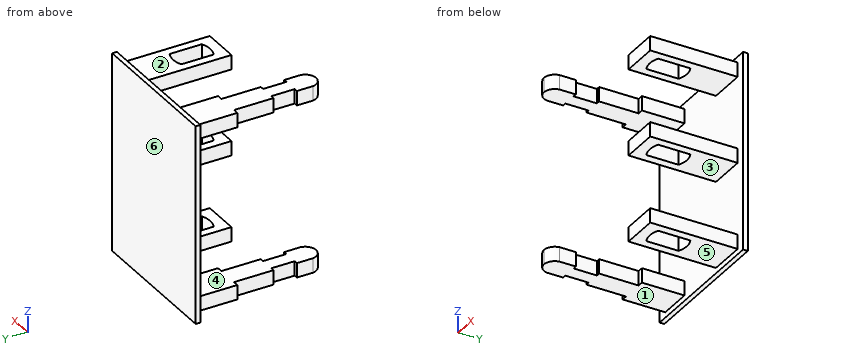
Autodesk Inventor part; units mm, degrees
ref_plane "terminal_to_body_XY" through (0, 0, 0) normal (0, 1, 0) x (1, 0, 0)
ref_plane "terminal_to_body_YZ" through (0, 0, 0) normal (1, 0, 0) x (0, 0, -1)
ref_plane "terminal_to_body_ZX" through (0, 0, 0) normal (0, 0, -1) x (0, 1, 0)
sketch "Sketch_1" plane through (0, 0.762, 0) normal (0, 1, 0) x (1, 0, 0)
  line L0 (-6.096, 6.096) -> (-6.096, -6.096)
  line L1 (-6.096, -6.096) -> (6.096, -6.096)
  line L2 (6.096, -6.096) -> (6.096, 6.096)
  line L3 (6.096, 6.096) -> (-6.096, 6.096)
extrude "Extrusion1" add sketch "Sketch_1" along normal blind 0.254
sketch "Sketch_2" plane through (0, 0, 0) normal (0, 0, 1) x (1, 0, 0)
  line L0 (1.397, -3.9878) -> (3.4036, -3.9878)
  line L1 (3.4036, -3.9878) -> (3.4036, 0.762)
  line L2 (3.4036, 0.762) -> (1.397, 0.762)
  line L3 (1.397, 0.762) -> (1.397, -3.9878)
  line L4 (1.8542, -1.5367) -> (1.8542, -3.2893)
  arc A0 (1.8542, -3.2893) -> (2.9464, -3.2893) centre (2.4003, -2.1787) ccw
  line L5 (2.9464, -3.2893) -> (2.9464, -1.5367)
  arc A1 (2.9464, -1.5367) -> (1.8542, -1.5367) centre (2.4003, -2.6473) ccw
extrude "Extrusion2" add sketch "Sketch_2" along normal mid plane 10.1854
sketch "Sketch_3" plane through (0, 0, 0) normal (0, 0, 1) x (1, 0, 0)
  line L0 (-3.2893, -1.5494) -> (-2.9845, -1.5494)
  line L1 (-2.9845, -1.5494) -> (-2.9845, -3.6957)
  line L2 (-2.9845, -3.6957) -> (-2.7813, -3.6957)
  line L3 (-2.7813, -3.6957) -> (-2.7813, -4.9657)
  line L4 (-2.7813, -4.9657) -> (-2.9845, -4.9657)
  line L5 (-2.9845, -4.9657) -> (-2.9845, -5.842)
  arc A0 (-2.9845, -5.842) -> (-1.8161, -5.842) centre (-2.4003, -5.7601) ccw
  line L6 (-1.8161, -5.842) -> (-1.8161, -4.9657)
  line L7 (-1.8161, -4.9657) -> (-2.0193, -4.9657)
  line L8 (-2.0193, -4.9657) -> (-2.0193, -3.6957)
  line L9 (-2.0193, -3.6957) -> (-1.8161, -3.6957)
  line L10 (-1.8161, -3.6957) -> (-1.8161, -1.5494)
  line L11 (-1.8161, -1.5494) -> (-1.5113, -1.5494)
  line L12 (-1.5113, -1.5494) -> (-1.5113, 0.762)
  line L13 (-1.5113, 0.762) -> (-3.2893, 0.762)
  line L14 (-3.2893, 0.762) -> (-3.2893, -1.5494)
extrude "Extrusion3" add sketch "Sketch_3" along normal mid plane 10.1854
sketch "Sketch_4" plane through (0, 0, 0) normal (1, 0, 0) x (0, 1, 0)
  line L0 (-7.1882, 5.9756) -> (-7.1882, -5.9196)
  line L1 (-7.1882, -5.9196) -> (0.762, -5.9196)
  line L2 (0.762, -5.9196) -> (0.762, -5.0927)
  line L3 (0.762, -5.0927) -> (-6.35, -5.0927)
  line L4 (-6.35, -5.0927) -> (-6.35, -4.3053)
  line L5 (-6.35, -4.3053) -> (0.762, -4.3053)
  line L6 (0.762, -4.3053) -> (0.762, -0.3937)
  line L7 (0.762, -0.3937) -> (-6.35, -0.3937)
  line L8 (-6.35, -0.3937) -> (-6.35, 0.3937)
  line L9 (-6.35, 0.3937) -> (0.762, 0.3937)
  line L10 (0.762, 0.3937) -> (0.762, 4.3053)
  line L11 (0.762, 4.3053) -> (-6.35, 4.3053)
  line L12 (-6.35, 4.3053) -> (-6.35, 5.0927)
  line L13 (-6.35, 5.0927) -> (0.762, 5.0927)
  line L14 (0.762, 5.0927) -> (0.762, 5.9756)
  line L15 (0.762, 5.9756) -> (-7.1882, 5.9756)
extrude "Extrusion4" cut sketch "Sketch_4" along normal mid plane 10.16
sketch "Sketch_19" plane through (0, 0.762, 0) normal (0, 1, 0) x (1, 0, 0)
  line L0 (-6.096, 6.096) -> (-6.096, -6.096)
  line L1 (-6.096, -6.096) -> (6.096, -6.096)
  line L2 (6.096, -6.096) -> (6.096, 6.096)
  line L3 (6.096, 6.096) -> (-6.096, 6.096)
  line L4 (-3.81, -5.4076) -> (3.9067, -5.4076)
  line L5 (3.9067, -5.4076) -> (3.9067, 5.3855)
  line L6 (3.9067, 5.3855) -> (-3.81, 5.3855)
  line L7 (-3.81, 5.3855) -> (-3.81, -5.4076)
extrude "Extrusion5" cut sketch "Sketch_19" along normal blind 2.54
sketch "Sketch_24" plane through (0, 0, 0) normal (0, 0, 1) x (1, 0, 0)
  line L0 (-8.7503, -7.62) -> (-1.2573, -7.62)
  line L1 (-1.2573, -7.62) -> (-1.2573, 0.762)
  line L2 (-1.2573, 0.762) -> (-8.7503, 0.762)
  line L3 (-8.7503, 0.762) -> (-8.7503, -7.62)
extrude "Extrusion6" cut sketch "Sketch_24" along normal mid plane 2.54
ref_plane "terminal_to_body_XY" through (0, 0, 0) normal (0, 1, 0) x (1, 0, 0)
ref_plane "terminal_to_body_YZ" through (0, 0, 0) normal (1, 0, 0) x (0, 0, -1)
ref_plane "terminal_to_body_ZX" through (0, 0, 0) normal (0, 0, -1) x (0, 1, 0)
properties part number "M211LCW01-terminals"
The listing builds one solid part. Answer for the finished solid, in the listing's coordinates (mm). Face numbers are marked on the shaded views. A direction names the side the tool comes from. Coordinates: 2 decimals unless noted, no trailing zeros. Loops run counter-clockwise (first coordinate to the right, second up) from the corner with the lowest first, then second, coordinate; pieces in that order, holes last. Notation, with made-up numbers: (61.5, 31.25) -> (69.5, 31.25) arc R28 cw to (69.5, 52.25) -> close; hole circle Ø7 at (-35.75, 8). An arc over 180 degrees is marked (long way). Return JSON: item names as keys, results as strings. Group by question number.
(1) A cutting plane is placed at B-B on y = -4.25. Write down the section's boundary in (x, z).
(2) A cutting plane is placed at D-D on y = -1.25. Write down the section's boundary in (x, z).
(3) A cutting plane is placed at A-A on y = -2.5. Count the separate pieces of the cut face and the enclosed holes in it, and give its area (3 significant figures).
(4) Given pin 1 Ø1.5 at (y, z) = (-1, 3.5) entering from -X; pin 2 Ø0.6 at (y, z) = (-1.5, 0) entering from +X; pin 3 Ø2 at (x, y) = (3, -2.5) entering from -Z; pin 4 Ø0.6 at (y, z) = (-3, -5) entering from -X, each flat-ended and moving along its own axis, determine where each tip first touches the part or whether it passes through.
(5) Determine the mould class of the marked faces 4, 5 and 6 for opening direction Z: released by +Z, released by -Z, zero draft, split by the parting line, or undercut.
(6) Find the intervals of material crossed by probe 1 along Z at (x, y) = (1.5, -3.5); probe 2 along Z at (x, y) = (-3, -0.5); probe 3 along Y at (x, z) = (0, 0.5), in increasing order. Write a range as from..to.
(7) Which of the six approach directions +Z, -Z, +X, -X, +Y, -Y give full straight-line access (tool end or side, diameter ignored) to the marked faces 1, 2 and 3?
The answers:
{
 "1": {"outline": "(-2.78, -5.09) -> (-2.02, -5.09) -> (-2.02, -4.31) -> (-2.78, -4.31) -> close; (-2.78, 4.31) -> (-2.02, 4.31) -> (-2.02, 5.09) -> (-2.78, 5.09) -> close"},
 "2": {"outline": "(-3.29, -5.09) -> (-1.51, -5.09) -> (-1.51, -4.31) -> (-3.29, -4.31) -> close; (-3.29, 4.31) -> (-1.51, 4.31) -> (-1.51, 5.09) -> (-3.29, 5.09) -> close; (1.4, -5.09) -> (3.4, -5.09) -> (3.4, -4.31) -> (1.4, -4.31) -> close; (1.4, -0.39) -> (3.4, -0.39) -> (3.4, 0.39) -> (1.4, 0.39) -> close; (1.4, 4.31) -> (3.4, 4.31) -> (3.4, 5.09) -> (1.4, 5.09) -> close"},
 "3": {"separate pieces": "8", "enclosed holes": "0", "area": "4.00 mm^2"},
 "4": {"pin 1": "passes through", "pin 2": "stops at x = 3.4", "pin 3": "stops at z = -5.09", "pin 4": "stops at x = -2.98"},
 "5": {"face 4": "undercut", "face 5": "released by -Z", "face 6": "zero draft"},
 "6": {"probe 1": "z = -5.09..-4.31, -0.39..0.39, 4.31..5.09", "probe 2": "z = -5.09..-4.31, 4.31..5.09", "probe 3": "y = 0.76..1.02"},
 "7": {"face 1": "-Z, +X, -X, -Y", "face 2": "+Z, +X, -X, -Y", "face 3": "+X, -X, -Y"}
}
